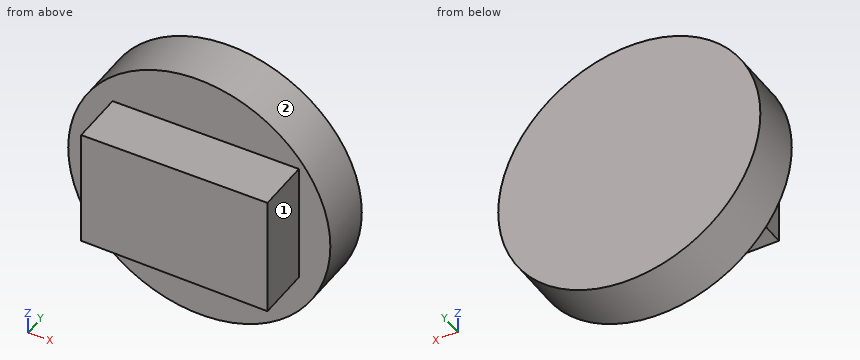
from build123d import *

# Parameters (mm, degrees)
F1_DEPTH = 0.0254
F3_R     = 62.6980879208
F4_DEPTH = 25.4
F6_DEPTH = 25.4


with BuildPart() as f1:
    # F0 (on Front) → F1 (new body)
    with BuildSketch(Plane.XZ):
        Polygon((47.9219257832, 17.5153240561), (-52.4058490992, 55.9089146554), (-52.4058490992, -55.068179965), align=None)
    extrude(amount=F1_DEPTH)


with BuildPart() as f4:
    # F3 (on Front) → F4 (new body)
    with BuildSketch(Plane.XZ):
        Circle(F3_R)
    extrude(amount=F4_DEPTH)

    # F5 (on face) → F6 (join)
    with BuildSketch(Plane.XZ.offset(25.4)):
        Polygon((47.6416796446, 35.1707711816), (-41.4762869477, 33.769544214), (-41.4762869477, -22.8399839252), (47.6416796446, -22.8399839252), align=None)
    extrude(amount=F6_DEPTH)


solid = f4.part
Work out the finished part from the listing and answer in its coordinate system (mm). Face numbers are marked on the shaded views. A direction names the side the tool comes from. Round coordinates to 2 decimals unless told otherwise and drop trailing zeros. Order: outer loops, then holes, each group sorted by start corner. A loop starts at its lowest first (then second) coordinate and runs counter-clockwise, first axis right, second up. Notation, with made-up numbers: M 54,60 L 101,60 A20 ccw 101,87 Z; hole C 83.5,-8 d8. An arc over 180 degrees is marked long. Put each result on its own line as item: value. Start each with the question number.
Q1. Section B-B, the plane x = 11 is taken. Write down the section's boundary in (y, z).
Q2. Flat-ended cylindrical pins translate along their axes: pin 1 (10 mm diameter, centred on x = 32.5, z = -36.5, fed in from -Y); pin 2 (12.5 mm diameter, centred on y = -36, z = 13.5, fed in from +X); pin 3 (10 mm diameter, centred on y = -8.5, z = -27.5, fed in from +X); pin 4 (10 mm diameter, centred on y = -34, z = -44.5, fed in from +X). Find the tip coordinate at first contact, or state that the pin passes through.
Q3. Section D-D, the plane y = -7 is taken. Write down the section's boundary in (x, z).
Q4. A tool of negligible diameter and unlimited length cuts with its end or side. For the marked faces 1 and 2, from which of +Z, -Z, +X, -X, +Y, -Y can it reach the whole face along a straight path? Write none if from no direction.
Q5. Section A-A, the plane z = 0 is taken. Write down the section's boundary in (x, y).
Q6. Section C-C, the plane y = -45.5 is taken. Write down the section's boundary in (x, z).
Q7. Straight lines are drawn through the part: L1, parallel to Y at x = 0, z = 56.5; L2, parallel to Z at x = 46, y = -41; L3, parallel to Z at x = 20, y = -15.5. For each, find the intervals that lie inside material, in ascending order. Write a range as [from, to].
Findings below:
1. outline: M -50.8,-22.84 L -25.4,-22.84 L -25.4,-61.73 L 0,-61.73 L 0,61.73 L -25.4,61.73 L -25.4,34.59 L -50.8,34.59 Z
2. pin 1: stops at y = -25.4
2. pin 2: stops at x = 47.64
2. pin 3: stops at x = 58.52
2. pin 4: passes through
3. outline: C 0,0 d125.4
4. face 1: +Z, -Z, +X, -Y
4. face 2: +Y, -Y
5. outline: M -62.7,-25.4 L -41.48,-25.4 L -41.48,-50.8 L 47.64,-50.8 L 47.64,-25.4 L 62.7,-25.4 L 62.7,0 L -62.7,0 Z
6. outline: M -41.48,-22.84 L 47.64,-22.84 L 47.64,35.17 L -41.48,33.77 Z
7. L1: y = [-25.4, 0]
7. L2: z = [-22.84, 35.14]
7. L3: z = [-59.42, 59.42]
